Can you work these out from the model? Positions are in its coordinate system, mm. Face numbers are marked on the shaded views. Give positions to 0.01 mm unless a question says otherwise; leave off trailing zeros. Order: outer loops, then holes, each group sorted by start corner. A loop starts at its lowest first (then second) coordinate and runs counter-clockwise, first axis right, second up.
```python
from build123d import *

# Parameters (mm, degrees)
SKETCH1_R           = 10
SKETCH1_R_2         = 2
SKETCH1_R_3         = 1
BOSS_EXTRUDE1_DEPTH = 1.5
SKETCH2_R           = 5
BOSS_EXTRUDE2_DEPTH = 50


with BuildPart() as part:
    # Sketch1 → Boss-Extrude1 (new body)
    # profile 1 of 2: a face of its own
    with BuildSketch(Plane(origin=(0, 0, 0), x_dir=(1, 0, 0), z_dir=(0, 1, 0))):
        with Locations(Location((0, 0, 0), (0, 0, 270))):
            Circle(SKETCH1_R)
        Circle(SKETCH1_R_2, mode=Mode.SUBTRACT)
        with Locations(Location((0, -7, 0), (0, 0, 270))):
            Circle(SKETCH1_R_3, mode=Mode.SUBTRACT)
        with Locations(Location((7, 0, 0), (0, 0, 270))):
            Circle(SKETCH1_R_3, mode=Mode.SUBTRACT)
        with Locations(Location((0, 7, 0), (0, 0, 270))):
            Circle(SKETCH1_R_3, mode=Mode.SUBTRACT)
        with Locations(Location((-7, 0, 0), (0, 0, 270))):
            Circle(SKETCH1_R_3, mode=Mode.SUBTRACT)
    # profile 2 of 2: a face of its own
    with BuildSketch(Plane(origin=(0, 0, 0), x_dir=(1, 0, 0), z_dir=(0, 1, 0))):
        Circle(SKETCH1_R_2)
    boss_extrude1 = extrude(amount=BOSS_EXTRUDE1_DEPTH)

    # Sketch2 → Boss-Extrude2 (add)
    with BuildSketch(Plane(origin=(0, 1.5, 0), x_dir=(1, 0, 0), z_dir=(0, 1, 0))):
        with Locations(Location((0, 0, 0), (0, 0, 270))):
            Circle(SKETCH2_R)
    extrude(amount=BOSS_EXTRUDE2_DEPTH)

    # Mirror1: Boss-Extrude1 across plane
    add(boss_extrude1.mirror(Plane.ZX.offset(26.5)))


solid = part.part
```
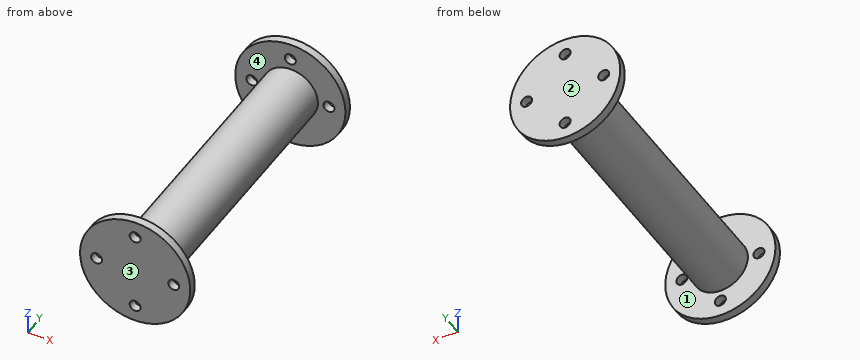
1) We'd pull the mould along Y, two halves only. Please class the marked faces 1, 2, 3 and 4: +Y half, -Y half, draft (parallel to the pull), parting line (faces both ways), or undercut.
2) If I drill on line 1 (X direction, y = 52, z = 0); line 2 (Y direction, x = 6, z = -6.25); line 3 (X direction, y = 52.55, z = -7), over which ranges is the centre line in solid material (lowest first)?
3) Suppose I cut it at B-B (z = -7). Please give me the cut outline in (x, y).
4) I'm going to push flat-ended pins straight in: pin 1 Ø3 at (y, z) = (18.5, 1) entering from +X; pin 2 Ø1.6 at (x, z) = (7, 0) entering from -Y; pin 3 Ø1.5 at (y, z) = (21.5, 2) entering from +X; pin 4 Ø5 at (x, y) = (-5.5, 47) entering from +Z. Where does each tip first touch, or does it pass through?
5) Suppose I cut it at D-D (z = 3.5). Please give me the cut outline in (x, y), and give its area (3 significant figures).
6) Suppose I cut it at C-C (x = 6.5). Please give me the cut outline in (y, z), and give its area (3 significant figures).
7) Suppose I cut it at A-A (x = 0). Please give me the cut outline in (y, z), and give its area (3 significant figures).
Results:
1. face 1: undercut
1. face 2: +Y half
1. face 3: -Y half
1. face 4: undercut
2. line 1: x = -10 to -8, -6 to 6, 8 to 10
2. line 2: y = 0 to 1.5, 51.5 to 53
2. line 3: x = -7.14 to -1, 1 to 7.14
3. outline: (-7.14, 0) - (-1, 0) - (-1, 1.5) - (-7.14, 1.5) - close; (-7.14, 51.5) - (-1, 51.5) - (-1, 53) - (-7.14, 53) - close; (1, 0) - (7.14, 0) - (7.14, 1.5) - (1, 1.5) - close; (1, 51.5) - (7.14, 51.5) - (7.14, 53) - (1, 53) - close
4. pin 1: stops at x = 5
4. pin 2: passes through
4. pin 3: stops at x = 4.84
4. pin 4: stops at z = 4
5. outline: (-9.37, 0) - (9.37, 0) - (9.37, 1.5) - (3.57, 1.5) - (3.57, 51.5) - (9.37, 51.5) - (9.37, 53) - (-9.37, 53) - (-9.37, 51.5) - (-3.57, 51.5) - (-3.57, 1.5) - (-9.37, 1.5) - close
5. area: 413 mm2
6. outline: (0, -7.6) - (1.5, -7.6) - (1.5, -0.87) - (0, -0.87) - close; (0, 0.87) - (1.5, 0.87) - (1.5, 7.6) - (0, 7.6) - close; (51.5, -7.6) - (53, -7.6) - (53, -0.87) - (51.5, -0.87) - close; (51.5, 0.87) - (53, 0.87) - (53, 7.6) - (51.5, 7.6) - close
6. area: 40.4 mm2
7. outline: (0, -10) - (1.5, -10) - (1.5, -8) - (0, -8) - close; (0, -6) - (1.5, -6) - (1.5, -5) - (51.5, -5) - (51.5, -6) - (53, -6) - (53, 6) - (51.5, 6) - (51.5, 5) - (1.5, 5) - (1.5, 6) - (0, 6) - close; (0, 8) - (1.5, 8) - (1.5, 10) - (0, 10) - close; (51.5, -10) - (53, -10) - (53, -8) - (51.5, -8) - close; (51.5, 8) - (53, 8) - (53, 10) - (51.5, 10) - close
7. area: 548 mm2
